Here's how the part is built. I have some questions about the finished solid (model axes, mm). A direction names the side the tool comes from. Give positions to 0.01 mm unless a question says otherwise; leave off trailing zeros. Loops run counter-clockwise (first coordinate to the right, second up) from the corner with the lowest first, then second, coordinate; pieces in that order, holes last. Notation, with made-up numbers: (55, 16.5) -> (92, 16.5) arc R17 cw to (92, 41.5) -> close; hole circle Ø11 at (21, -10.75). An arc over 180 degrees is marked (long way). Answer in a Markdown table with one row per item. Add a question column.
Item 1: If we section it at A-A (x = 6): Write out the boundary of the cut face in (y, z), then the cut area to 3 significant figures.
Item 2: If I drill on line 1 (Y direction, x = 3.5, z = 1.6); line 2 (X direction, y = -7, z = 2), over which ranges is the centre line in solid material (lowest first)?
Item 3: Which directions (+Z, -Z, +X, -X, +Y, -Y) give clear straight access to the entire face, cutting with the end or side of a thin tool? Please do faces 1 (the face through (11, 0, 3.3)), 2 (the face through (8.7, 0, 3)), 3 (the face through (0, 7.7, 1)).
Item 4: We'd pull the mould along X, two halves only. Please class faces 4 (the face through (-7.7, 0, 1)), 5 (the face through (17.5, 0, 2)), 6 (the face through (-18, 18, 0.206)), 7 (the face through (7.7, 0, 1)): released by +X, released by -X, zero draft, split by the parting line, or undercut.
Item 5: If we section it at D-D (y = 16): Write out the boundary of the cut face in (x, z), then the cut area to 3 significant figures.
Item 6: If we section it at C-C (x = 20.5): Write out the boundary of the cut face in (y, z), then the cut area to 3 significant figures.
Item 7: For P1, Ø0.7, axis at y = 0.5, z = 3, coming from the -X side; P2, Ø0.6, axis at y = 0, z = 0.5, coming from the +X side; P3, Ø1, axis at x = -9, z = 0.5, coming from the -Y side, each with a flat end and sliding along its axis, tell me the tip position at first contact or that it passes through.
```python
from build123d import *

# Parameters (mm, degrees)
F0_W     = 17.4
F0_H     = 17.4
F0_W_2   = 15.4
F0_H_2   = 15.4
F5_DEPTH = 1.9
F0_W_3   = 35
F0_H_3   = 35
F1_DEPTH = 1.9
F2_DEPTH = 1.4
F3_R     = 7.5
F4_DEPTH = 0.2064


with BuildPart() as f5:
    # F0 (on Top) → F5 (new body)
    with BuildSketch(Plane.XY):
        Rectangle(F0_W, F0_H)
        Rectangle(F0_W_2, F0_H_2, mode=Mode.SUBTRACT)
    extrude(amount=F5_DEPTH)



with BuildPart() as f1:
    # F0 (on Top) → F1 (new body, through all)
    with BuildSketch(Plane.XY):
        Rectangle(F0_W_3, F0_H_3)
        Rectangle(F0_W, F0_H, mode=Mode.SUBTRACT)
    extrude(amount=F1_DEPTH)


with BuildPart() as f5_1:
    add(f5.part)
    # F2 (add): a face of the model
    f2_faces = [f1.part.faces().sort_by_distance(p)[0] for p in [
        (17.0050252532, 0, 1.9),
    ]]

    add(f1.part)  # F2 merges F1
    extrude(f2_faces, amount=F2_DEPTH)

    # F3 (on Top) → F4 (join)
    with BuildSketch(Plane.XY):
        with Locations((17.5, 17.5)):
            Circle(F3_R)
        with Locations((-17.5, 17.5)):
            Circle(F3_R)
        with Locations((-17.5, -17.5)):
            Circle(F3_R)
        with Locations((17.5, -17.5)):
            Circle(F3_R)
    extrude(amount=F4_DEPTH)


solid = f5_1.part
```
Recorded:
| question | item | result |
|---|---|---|
| 1 | outline | (-17.5, 0) -> (-7.7, 0) -> (-7.7, 1.9) -> (-8.7, 1.9) -> (-8.7, 3.3) -> (-17.5, 3.3) -> close; (7.7, 0) -> (17.5, 0) -> (17.5, 3.3) -> (8.7, 3.3) -> (8.7, 1.9) -> (7.7, 1.9) -> close |
| 1 | area | 61.9 mm^2 |
| 2 | line 1 | y = -17.5 to -7.7, 7.7 to 17.5 |
| 2 | line 2 | x = -17.5 to -8.7, 8.7 to 17.5 |
| 3 | face 1 | +Z, +X, -X, +Y, -Y |
| 3 | face 2 | +Z |
| 3 | face 3 | +Z, -Z |
| 4 | face 4 | undercut |
| 4 | face 5 | released by +X |
| 4 | face 6 | zero draft |
| 4 | face 7 | undercut |
| 5 | outline | (-24.85, 0) -> (24.85, 0) -> (24.85, 0.21) -> (17.5, 0.21) -> (17.5, 3.3) -> (-17.5, 3.3) -> (-17.5, 0.21) -> (-24.85, 0.21) -> close |
| 5 | area | 119 mm^2 |
| 6 | outline | (-24.37, 0) -> (-10.63, 0) -> (-10.63, 0.21) -> (-24.37, 0.21) -> close; (10.63, 0) -> (24.37, 0) -> (24.37, 0.21) -> (10.63, 0.21) -> close |
| 6 | area | 5.68 mm^2 |
| 7 | P1 | stops at x = -17.5 |
| 7 | P2 | stops at x = 17.5 |
| 7 | P3 | stops at y = -17.5 |
